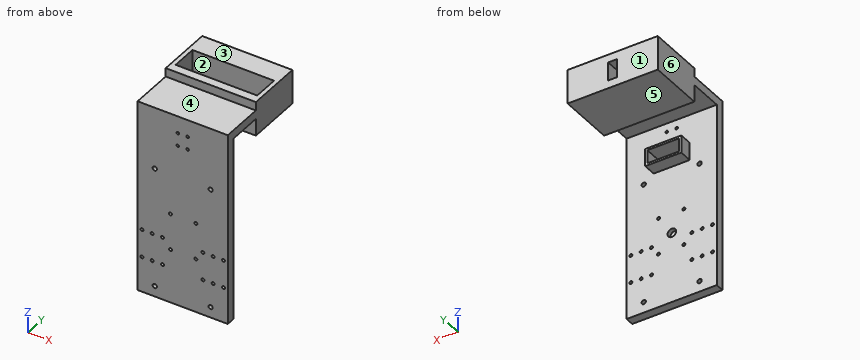
Autodesk Inventor part; units mm, degrees
ref_plane "YZ Plane" through (0, 0, 0) normal (1, 0, 0) x (0, 1, 0)
ref_plane "XZ Plane" through (0, 0, 0) normal (0, 1, 0) x (-1, 0, 0)
ref_plane "XY Plane" through (0, 0, 0) normal (0, 0, 1) x (1, 0, 0)
sketch "Boceto1" plane through (0, 0, 0) normal (1, 0, 0) x (0, 1, 0)
  line L0 (10, 225) -> (-10, 225)
  line L1 (-10, 225) -> (-10, -225)
  line L2 (-10, -225) -> (10, -225)
  line L3 (10, -225) -> (10, 225)
  line L4 (10, 225) -> (-10, -225) construction
  line L5 (-10, 225) -> (10, -225) construction
  point P0 (0, 0)
  dimension "d0" = 20
  dimension "d1" = 450
extrude "Extrusión1" add sketch "Boceto1" along normal blind 210
sketch "Boceto2" plane through (0, 10, 225) normal (0, 1, 0) x (1, 0, 0)
  line L0 (0, 0) -> (0, 450)
  line L1 (210, 0) -> (210, 450)
  line L2 (0, 0) -> (210, 0)
  line L3 (210, 0) -> (210, 20)
  line L4 (210, 20) -> (0, 20)
  line L5 (0, 20) -> (0, 0)
  point P0 (0, 225)
  dimension "d4" = 20
extrude "Extrusión2" add sketch "Boceto2" along normal blind 80
sketch "Boceto3" plane through (0, 90, 225) normal (0, 1, 0) x (1, 0, 0)
  line L0 (0, 0) -> (210, 0)
  line L1 (0, 0) -> (210, 0)
  line L2 (210, 0) -> (210, -20)
  line L3 (210, -20) -> (0, -20)
  line L4 (0, -20) -> (0, 0)
  line L5 (0, 0) -> (210, 0)
  line L6 (210, 0) -> (210, 60)
  line L7 (210, 60) -> (0, 60)
  line L8 (0, 60) -> (0, 0)
  point P0 (0, 225)
  dimension "d7" = 20
  dimension "d8" = 210
  dimension "d9" = 60
extrude "Extrusión3" add sketch "Boceto3" along normal blind 130
sketch "Boceto4" plane through (0, 90, 245) normal (0, 0, 1) x (1, 0, 0)
  line L0 (10, 80) -> (200, 80)
  line L1 (200, 80) -> (200, 20)
  line L2 (200, 20) -> (10, 20)
  line L3 (10, 20) -> (10, 80)
  point P0 (0, -90)
  point P1 (0, 130)
  point P2 (210, 0)
  dimension "d12" = 190
  dimension "d13" = 60
extrude "Extrusión4" cut sketch "Boceto4" against normal blind 60
sketch "Boceto5" plane through (0, 220, 225) normal (0, 1, 0) x (1, 0, 0)
  line L0 (94.5, -1.5) -> (115.5, -1.5)
  line L1 (115.5, -1.5) -> (115.5, 41.5)
  line L2 (115.5, 41.5) -> (94.5, 41.5)
  line L3 (94.5, 41.5) -> (94.5, -1.5)
  line L4 (94.5, -1.5) -> (115.5, 41.5) construction
  line L5 (115.5, -1.5) -> (94.5, 41.5) construction
  point P0 (0, 225)
  point P1 (105, 20)
  dimension "d18" = 21
  dimension "d19" = 43
extrude "Extrusión5" cut sketch "Boceto5" against normal blind 43
sketch "Boceto6" plane through (0, 10, -225) normal (0, 1, 0) x (1, 0, 0)
  circle A0 centre (40, -305) radius 5
  circle A1 centre (40, -25) radius 5
  circle A2 centre (170, -305) radius 5
  circle A3 centre (170, -25) radius 5
  line L0 (0, -470) -> (210, -470)
  line L1 (0, 0) -> (210, 0)
  line L2 (0, 0) -> (0, -430)
  line L3 (210, 0) -> (210, -430)
  point P0 (0, -225)
  dimension "d23" = 10
  dimension "d24" = 10
  dimension "d25" = 10
  dimension "d26" = 10
  dimension "d27" = 165
  dimension "d28" = 25
  dimension "d29" = 25
  dimension "d30" = 165
  dimension "d31" = 40
  dimension "d32" = 40
  dimension "d33" = 40
  dimension "d34" = 40
extrude "Extrusión6" cut sketch "Boceto6" against normal blind 43
sketch "Boceto7" plane through (0, 10, -225) normal (0, 1, 0) x (1, 0, 0)
  line L0 (0, 0) -> (210, 0)
  line L1 (0, 0) -> (210, 0)
  line L2 (210, 0) -> (105, 0)
  line L3 (210, -390) -> (0, -390)
  line L4 (105, -390) -> (105, 0)
  circle A0 centre (40, -305) radius 5
  circle A1 centre (40, -25) radius 5
  line L5 (40, -305) -> (40, -25)
  line L6 (40, -165) -> (169.1036, -165)
  circle A2 centre (104.5518, -165) radius 10
  point P0 (0, -225)
  dimension "d44" = 20
extrude "Extrusión7" cut sketch "Boceto7" against normal blind 10 contours A2 L6 L4 | L4 L6 A2 | L6 A2 L4 | L4 A2 L6
sketch "Boceto8" plane through (0, 10, -225) normal (0, 1, 0) x (1, 0, 0)
  circle A0 centre (104.5518, -165) radius 10
  circle A1 centre (135.5518, -211) radius 3.5
  line L0 (104.5518, -165) -> (126.1125, -165)
  circle A2 centre (135.5518, -126) radius 3.5
  circle A3 centre (76.5518, -126) radius 3.5
  circle A4 centre (76.5518, -211) radius 3.5
  point P0 (0, -225)
  dimension "d51" = 7
  dimension "d52" = 7
  dimension "d54" = 7
extrude "Extrusión8" cut sketch "Boceto8" against normal blind 20 contours A1 | A2 | A3 | A4
sketch "Boceto9" plane through (0, 10, -225) normal (0, 1, 0) x (1, 0, 0)
  line L0 (0, -430) -> (210, -430)
  line L1 (0, -430) -> (210, -430)
  circle A0 centre (93.5, -410) radius 3
  line L2 (210, -430) -> (0, -430)
  circle A1 centre (116.5, -410) radius 3
  circle A2 centre (93.5, -380) radius 3
  circle A3 centre (116.5, -380) radius 3
  point P0 (0, -225)
  dimension "d59" = 20
  dimension "d64" = 20
  dimension "d65" = 30
  dimension "d66" = 30
extrude "Extrusión9" cut sketch "Boceto9" against normal blind 20
sketch "Boceto10" plane through (0, 10, -225) normal (0, 1, 0) x (1, 0, 0)
  line L0 (0, -430) -> (210, -430)
  line L1 (68, -358.4637) -> (142, -358.4637)
  line L2 (142, -358.4637) -> (68, -358.4637)
  line L3 (68, -358.4637) -> (68, -327.4637)
  line L4 (68, -327.4637) -> (142, -327.4637)
  line L5 (142, -327.4637) -> (142, -358.4637)
  line L6 (68, -358.4637) -> (142, -327.4637)
  line L7 (68, -327.4637) -> (142, -358.4637)
  line L8 (63, -363.4637) -> (147, -363.4637)
  line L9 (147, -363.4637) -> (147, -322.4637)
  line L10 (147, -322.4637) -> (63, -322.4637)
  line L11 (63, -322.4637) -> (63, -363.4637)
  line L12 (63, -363.4637) -> (147, -322.4637) construction
  line L13 (147, -363.4637) -> (63, -322.4637) construction
  point P0 (0, -225)
  point P1 (105, -342.9637)
  dimension "d68" = 74
  dimension "d69" = 31
  dimension "d70" = 84
  dimension "d71" = 41
extrude "Extrusión10" cut sketch "Boceto10" against normal blind 10 contours L6 L7 L1 | L3 L7 L6 | L7 L6 L5 | L4 L6 L7
sketch "Boceto11" plane through (0, 10, -225) normal (0, 1, 0) x (1, 0, 0)
  line L0 (142, -358.4637) -> (68, -358.4637)
  line L1 (68, -358.4637) -> (142, -327.4637)
  line L2 (68, -327.4637) -> (142, -327.4637)
  line L3 (142, -327.4637) -> (68, -327.4637)
  line L4 (142, -327.4637) -> (142, -358.4637)
  line L5 (68, -327.4637) -> (142, -358.4637)
  line L6 (63, -363.4637) -> (147, -363.4637)
  line L7 (147, -363.4637) -> (147, -322.4637)
  line L8 (147, -322.4637) -> (63, -322.4637)
  line L9 (63, -322.4637) -> (63, -363.4637)
  line L10 (63, -363.4637) -> (147, -322.4637) construction
  line L11 (147, -363.4637) -> (63, -322.4637) construction
  line L12 (68, -358.4637) -> (142, -358.4637)
  line L13 (142, -358.4637) -> (142, -327.4637)
  line L14 (142, -327.4637) -> (68, -327.4637)
  line L15 (68, -327.4637) -> (68, -358.4637)
  line L16 (68, -358.4637) -> (142, -327.4637) construction
  line L17 (142, -358.4637) -> (68, -327.4637) construction
  point P0 (0, -225)
  point P1 (105, -342.9637)
  dimension "d74" = 84
  dimension "d75" = 41
extrude "Extrusión11" add sketch "Boceto11" along normal blind 30
sketch "Boceto12" plane through (0, 10, -225) normal (0, 1, 0) x (1, 0, 0)
  circle A0 centre (10, -147.8334) radius 3.5
  line L0 (0, -155.4334) -> (68, -155.4334)
  line L1 (68, -155.4334) -> (68, -75.4334)
  line L2 (68, -75.4334) -> (0, -75.4334)
  line L3 (0, -75.4334) -> (0, -155.4334)
  line L4 (34, -155.4334) -> (34, -124.7606)
  circle A1 centre (34, -147.8334) radius 3.5
  circle A2 centre (58, -147.8334) radius 3.5
  line L5 (68, -115.4334) -> (56.8167, -115.4334)
  circle A3 centre (10, -83.0334) radius 3.5
  circle A4 centre (34, -83.0334) radius 3.5
  circle A5 centre (58, -83.0334) radius 3.5
  line L6 (0, 0) -> (210, 0)
  line L7 (105, 0) -> (105, -79.7219)
  circle A6 centre (200, -147.8334) radius 3.5
  line L8 (210, -155.4334) -> (142, -155.4334)
  line L9 (142, -155.4334) -> (142, -75.4334)
  line L10 (142, -75.4334) -> (210, -75.4334)
  line L11 (210, -75.4334) -> (210, -155.4334)
  line L12 (176, -155.4334) -> (176, -124.7606)
  circle A7 centre (176, -147.8334) radius 3.5
  circle A8 centre (152, -147.8334) radius 3.5
  line L13 (142, -115.4334) -> (153.1833, -115.4334)
  circle A9 centre (152, -83.0334) radius 3.5
  circle A10 centre (176, -83.0334) radius 3.5
  circle A11 centre (200, -83.0334) radius 3.5
  point P0 (0, -225)
  point P1 (210, -225)
  dimension "d78" = 7
  dimension "d79" = 68
  dimension "d80" = 80
  dimension "d81" = 7.6
  dimension "d82" = 10
  dimension "d83" = 7
extrude "Extrusión12" cut sketch "Boceto12" against normal blind 30 contours A0 | A1 L4 | L4 A1 | A2 | A3 | A4 | A5 | A6 | A7 L12 | L12 A7 | A8 | A9 | A10 | A11
sketch "Boceto13" plane through (0, 10, -225) normal (0, 1, 0) x (1, 0, 0)
  line L0 (0, 0) -> (0, -430)
  line L1 (0, -180) -> (209.4793, -180)
  line L2 (0, 0) -> (210, 0)
  line L3 (0, -450) -> (0, 0)
  line L4 (0, -270) -> (210, -270)
  line L5 (210, -450) -> (210, 0)
  line L6 (210, -430) -> (0, -430)
  line L7 (0, -450) -> (210, -450)
  point P0 (0, -225)
  dimension "d103" = 180
  dimension "d110" = 180
split_face "Dividir1"
properties part number "base"
Model file for the job. Use its own axes, mm. Face numbers are marked on the shaded views. A direction names the side the tool comes from. Give positions to 0.01 mm unless a question says otherwise; leave off trailing zeros. Loops run counter-clockwise (first coordinate to the right, second up) from the corner with the lowest first, then second, coordinate; pieces in that order, holes last. Notation, with made-up numbers: (-27, 59.25) - (17, 59.25) arc R11 ccw to (17, 72.25) - close; hole circle Ø11 at (88, 41). An arc over 180 degrees is marked (long way). One line per item, written item: value. Start each with the question number.
1. Slice it at C-C (y = 149). List the corners of the cut face in (x, z).
2. Probe L1, parallel to Z at x = 176, y = -5.25; L2, parallel to X at y = -2.5, z = -200; L3, parallel to Z at x = 103.5, y = 12. List the from-to ranges inside material, lowest first. Write a range as from..to.
3. Slice it at D-D (z = -109.5). List the corners of the cut face in (x, y), plus the area to 3 significant figures.
4. Slice it at A-A (x = 127). List the corners of the cut face in (y, z).
5. Which spindle directions (+Z, -Z, +X, -X, +Y, -Y) get a long thin tool onto all of the face, cutting with end or side? Do the marked faces 4, 5 and 6. Say none if no direction does.
6. Slice it at B-B (z = 115.5). List the corners of the cut face in (x, y), plus the area to 3 significant figures.
7. Pull direction Y, two halves, no side cores. Call the marked faces 1, 2 and 3: pulls with the +Y half, pulls with the -Y half, needs draft (parallel to the pull), parting line crosses it, or undercut.
8. Pin check, flat tips, straight feed: pin 1 (6.5 mm diameter, centred on x = 76.55, z = -14, fed in from -Y); pin 2 (9 mm diameter, centred on x = 34, z = -77.17, fed in from +Y); pin 3 (1.5 mm diameter, centred on x = 170.5, y = 157.5, fed in from +Z); pin 4 (6 mm diameter, centred on x = 86.5, y = 115.5, fed in from -Z). Stop position of each tip, or through.
Solution:
1. outline: (0, 165) - (210, 165) - (210, 245) - (200, 245) - (200, 185) - (10, 185) - (10, 245) - (0, 245) - close
2. L1: z = -225..-145.47, -138.47..-80.67, -73.67..225
2. L2: x = 0..35, 45..165, 175..210
2. L3: z = 97.46..102.46, 133.46..138.46, 205..225
3. outline: (0, -10) - (210, -10) - (210, 10) - (0, 10) - close
3. area: 4,200 mm^2
4. outline: (-10, -225) - (10, -225) - (10, 97.46) - (40, 97.46) - (40, 102.46) - (0, 102.46) - (0, 133.46) - (40, 133.46) - (40, 138.46) - (10, 138.46) - (10, 205) - (90, 205) - (90, 165) - (220, 165) - (220, 245) - (170, 245) - (170, 185) - (110, 185) - (110, 245) - (90, 245) - (90, 225) - (-10, 225) - close
5. face 4: +Z, +X, -X, -Y
5. face 5: -Z, +X, -X, +Y
5. face 6: +Z, -Z, -X, +Y, -Y
6. outline: (0, -10) - (210, -10) - (210, 10) - (147, 10) - (147, 40) - (142, 40) - (142, 0) - (68, 0) - (68, 40) - (63, 40) - (63, 10) - (0, 10) - close
6. area: 3,760 mm^2
7. face 1: pulls with the +Y half
7. face 2: undercut
7. face 3: needs draft
8. pin 1: passes through
8. pin 2: stops at y = 10
8. pin 3: stops at z = 185
8. pin 4: stops at z = 165
